Read the model definition and answer for the solid it produces. Units are mm, in the model's axes. A direction names the side the tool comes from. Coordinates: 2 decimals unless noted, no trailing zeros. Loops run counter-clockwise (first coordinate to the right, second up) from the corner with the lowest first, then second, coordinate; pieces in that order, holes last. Notation, with made-up numbers: (-14, -18.5) - (32, -18.5) arc R12 cw to (32, -2.5) - close; hole circle Ø4 at (45, 4.25). An arc over 180 degrees is marked (long way). Use one line per item in the form item = value. Start each with the question number.
1) Each of these flat-tipped pins is pushed along its axis until it touches: P1, Ø5, axis at x = 55.5, y = 27.5, coming from the -Z side; P2, Ø13, axis at x = 40, y = 32.4, coming from the -Z side; P3, Ø3, axis at x = 8, y = 29, coming from the +Z side; P4, Ø1, axis at x = 48.5, z = 4.5, coming from the +Y side. Where does it stop, or does it pass through?
2) A cutting plane is placed at A-A (x = 10). Give the vertices of the cut face in (y, z), and give its area (3 significant figures).
3) The mould has two halves that part along Y. Classify faces 1 (the face through (39, 25, 12)), 2 (the face through (67.4, 30.1, 5.2)), 3 (the face through (39, 50, 6)): released by +Y, released by -Y, zero draft, split by the parting line, or undercut.
4) Which of the six approach directions +Z, -Z, +X, -X, +Y, -Y give full straight-line access (tool end or side, diameter ignored) to faces 4 (the face through (38, 38, 4.5)), 5 (the face through (72, 28, 10.45)), 6 (the face through (35.9, 36.2, 8.2))?
5) Consider line 1 (X direction, y = 48, z = 6); line 2 (Y direction, x = 10, z = 3); line 3 (Y direction, x = 16.5, z = 9.75). Determine where each line is inside the solid, lowest interval first.
6) A cutting plane is placed at C-C (y = 8.9). Give the vertices of the cut face in (x, z), and give its area (3 significant figures).
7) A cutting plane is placed at B-B (z = 1.25). Give the vertices of the cut face in (x, y).
8) A cutting plane is placed at D-D (x = 44.5). Give the vertices of the cut face in (y, z).
from build123d import *

# Parameters (mm, degrees)
CROQUIS1_W                       = 80
CROQUIS1_H                       = 50
CROQUIS1_R                       = 2.6
CROQUIS1_R_2                     = 5.59
CROQUIS1_R_3                     = 2.661703711
SALIENTE_EXTRUIR1_DEPTH          = 12
CROQUIS2_R                       = 4.6
CORTAR_EXTRUIR1_DEPTH            = 1.55
CROQUIS4_R                       = 8.05
CORTAR_EXTRUIR2_DEPTH            = 4.5
TALADRO_DE_MARGEN_PARA_M51_D     = 5.5
TALADRO_DE_MARGEN_PARA_M51_DEPTH = 10
TALADRO_DE_MARGEN_PARA_M51_TIP   = 1.652366702
TALADRO_DE_MARGEN_PARA_M52_D     = 5.5
TALADRO_DE_MARGEN_PARA_M52_DEPTH = 10
TALADRO_DE_MARGEN_PARA_M52_TIP   = 1.652366702


with BuildPart() as part:
    # Croquis1 → Saliente-Extruir1 (new body)
    with BuildSketch(Plane.XY):
        with Locations((40, 25)):
            Rectangle(CROQUIS1_W, CROQUIS1_H)
        with Locations((10, 30)):
            Circle(CROQUIS1_R, mode=Mode.SUBTRACT)
        with Locations((70, 30)):
            Circle(CROQUIS1_R, mode=Mode.SUBTRACT)
        with Locations((40, 32.4)):
            Circle(CROQUIS1_R_2, mode=Mode.SUBTRACT)
        with Locations((16.4, 8.9)):
            Circle(CROQUIS1_R_3, mode=Mode.SUBTRACT)
        with Locations((30, 10)):
            Circle(CROQUIS1_R, mode=Mode.SUBTRACT)
        with Locations((50, 10)):
            Circle(CROQUIS1_R, mode=Mode.SUBTRACT)
        with Locations((63.6, 8.9)):
            Circle(CROQUIS1_R, mode=Mode.SUBTRACT)
    extrude(amount=SALIENTE_EXTRUIR1_DEPTH)

    # Croquis2 → Cortar-Extruir1 (cut)
    with BuildSketch(Plane.XY.offset(12)):
        with Locations((10, 30)):
            Circle(CROQUIS2_R)
        with Locations((70, 30)):
            Circle(CROQUIS2_R)
        with Locations((30, 10)):
            Circle(CROQUIS2_R)
        with Locations((50, 10)):
            Circle(CROQUIS2_R)
    extrude(amount=-CORTAR_EXTRUIR1_DEPTH, mode=Mode.SUBTRACT)

    # Croquis4 → Cortar-Extruir2 (cut)
    with BuildSketch(Plane(origin=(0, 0, 0), x_dir=(-1, 0, 0), z_dir=(0, 0, -1))):
        with Locations((-40, 32.4)):
            Circle(CROQUIS4_R)
    extrude(amount=-CORTAR_EXTRUIR2_DEPTH, mode=Mode.SUBTRACT)

    # Taladro de margen para M51
    with Locations(Plane(origin=(30, 50, 6), x_dir=(0, 0, 1), z_dir=(0, 1, 0))):
        with Locations((0, 0)):
            Hole(TALADRO_DE_MARGEN_PARA_M51_D / 2, depth=TALADRO_DE_MARGEN_PARA_M51_DEPTH)
            with Locations((0, 0, -(TALADRO_DE_MARGEN_PARA_M51_DEPTH + TALADRO_DE_MARGEN_PARA_M51_TIP / 2))):  # 118° drill point
                Cone(0, TALADRO_DE_MARGEN_PARA_M51_D / 2, TALADRO_DE_MARGEN_PARA_M51_TIP, mode=Mode.SUBTRACT)

    # Taladro de margen para M52
    with Locations(Plane(origin=(50, 50, 6), x_dir=(0, 0, 1), z_dir=(0, 1, 0))):
        with Locations((0, 0)):
            Hole(TALADRO_DE_MARGEN_PARA_M52_D / 2, depth=TALADRO_DE_MARGEN_PARA_M52_DEPTH)
            with Locations((0, 0, -(TALADRO_DE_MARGEN_PARA_M52_DEPTH + TALADRO_DE_MARGEN_PARA_M52_TIP / 2))):  # 118° drill point
                Cone(0, TALADRO_DE_MARGEN_PARA_M52_D / 2, TALADRO_DE_MARGEN_PARA_M52_TIP, mode=Mode.SUBTRACT)


solid = part.part
Found:
q1.P1 = 0
q1.P2 = 4.5
q1.P3 = 10.45
q1.P4 = 39.92
q2.outline = (0, 0) - (27.4, 0) - (27.4, 10.45) - (25.4, 10.45) - (25.4, 12) - (0, 12) - close; (32.6, 0) - (50, 0) - (50, 12) - (34.6, 12) - (34.6, 10.45) - (32.6, 10.45) - close
q2.area = 531 mm^2
q3.face_1 = zero draft
q3.face_2 = undercut
q3.face_3 = released by +Y
q4.face_4 = -Z
q4.face_5 = +Z
q4.face_6 = +Z, -Z
q5.line_1 = 0 to 27.25, 32.75 to 47.25, 52.75 to 80
q5.line_2 = 0 to 27.4, 32.6 to 50
q5.line_3 = 0 to 6.24, 11.56 to 50
q6.outline = (0, 0) - (13.74, 0) - (13.74, 12) - (0, 12) - close; (19.06, 0) - (27.64, 0) - (27.64, 10.45) - (25.53, 10.45) - (25.53, 12) - (19.06, 12) - close; (32.36, 0) - (47.64, 0) - (47.64, 10.45) - (45.53, 10.45) - (45.53, 12) - (34.47, 12) - (34.47, 10.45) - (32.36, 10.45) - close; (52.36, 0) - (61, 0) - (61, 12) - (54.47, 12) - (54.47, 10.45) - (52.36, 10.45) - close; (66.2, 0) - (80, 0) - (80, 12) - (66.2, 12) - close
q6.area = 708 mm^2
q7.outline = (0, 0) - (80, 0) - (80, 50) - (0, 50) - close; hole circle Ø5.2 at (10, 30); hole circle Ø5.32 at (16.4, 8.9); hole circle Ø5.2 at (30, 10); hole circle Ø16.1 at (40, 32.4); hole circle Ø5.2 at (50, 10); hole circle Ø5.2 at (63.6, 8.9); hole circle Ø5.2 at (70, 30)
q8.outline = (0, 0) - (25.73, 0) - (25.73, 4.5) - (29.08, 4.5) - (29.08, 12) - (0, 12) - close; (35.72, 4.5) - (39.07, 4.5) - (39.07, 0) - (50, 0) - (50, 12) - (35.72, 12) - close
